Check sheet for the modelled part. Datum: model origin and axes. Units: mm. Face numbers are marked on the shaded views. A direction names the side the tool comes from. Give positions to 0.01 mm unless a question says otherwise; leave off trailing zeros. Order: outer loops, then holes, each group sorted by start corner. A loop starts at its lowest first (then second) coordinate and runs counter-clockwise, first axis right, second up. Notation, with made-up numbers: M 21.5,17 L 57.5,17 A11 ccw 57.5,32 Z; hole C 62,64.25 d8. An arc over 180 degrees is marked long. Return JSON: item names as keys, results as strings. Group by question number.
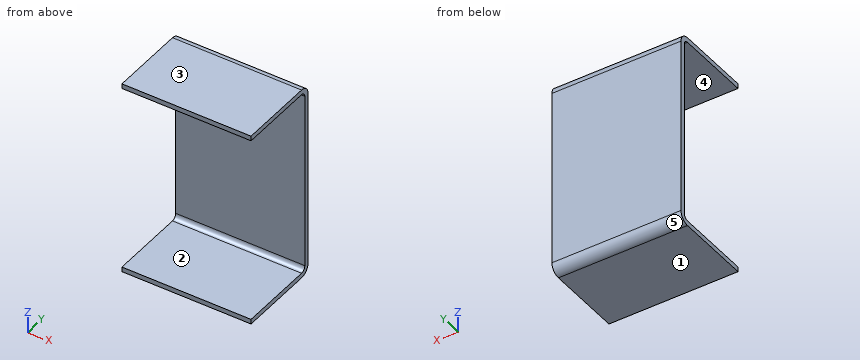
from build123d import *

# Parameters (mm, degrees)
EXTRUDE_1_DEPTH       = 40
SHEET_START           = -40
SHEET_METAL_1_DEPTH   = 80
SHEET_METAL_1_2_DEPTH = 80


# Read off the part's stored shape, not the designer's step: Преобразовать-Твердое тело1
with BuildPart() as part:
    # Sketch 1 → Вытянуть-Тонкостенный1 (new, symmetric)
    with BuildSketch(Plane(origin=(0, 0, 0), x_dir=(0, 0, -1), z_dir=(1, 0, 0))):
        Polygon((-58, -25), (-58, 25), (58, 25), (58, -25), (64, -25), (64, 31), (-64, 31), (-64, -25), align=None)
    extrude(amount=EXTRUDE_1_DEPTH, both=True)

    # Sheet Metal 1 outline → Sheet Metal 1 (cut)
    with BuildSketch(Plane.YZ.offset(SHEET_START)):
        with BuildLine():
            Line((-25, 64), (-25, 61))
            Line((-25, 61), (22, 61))
            ThreePointArc((22, 61), (26.242640687, 59.242640687), (28, 55))
            Line((28, 55), (28, -55))
            ThreePointArc((28, -55), (26.242640687, -59.242640687), (22, -61))
            Line((22, -61), (-25, -61))
            Line((-25, -61), (-25, -64))
            Line((-25, -64), (31, -64))
            Line((31, -64), (31, 64))
            Line((31, 64), (-25, 64))
        make_face()
    extrude(amount=SHEET_METAL_1_DEPTH, mode=Mode.SUBTRACT)

    # Sheet Metal 1 2 outline → Sheet Metal 1 2 (add)
    with BuildSketch(Plane.YZ.offset(SHEET_START)):
        with BuildLine():
            ThreePointArc((22, 58), (24.121320344, 57.121320344), (25, 55))
            Line((25, 55), (25, 58))
            Line((25, 58), (22, 58))
        make_face()
        with BuildLine():
            Line((25, -58), (25, -55))
            ThreePointArc((25, -55), (24.121320344, -57.121320344), (22, -58))
            Line((22, -58), (25, -58))
        make_face()
    extrude(amount=SHEET_METAL_1_2_DEPTH)


solid = part.part
1) Material ranges on line 1 along Z through (x, y) = (17, -18); line 2 along Y through (x, z) = (-11.5, -44); line 3 along Z through (x, y) = (-33.5, 26.5), recorded low to high.
2) Tool access check on the marked faces 4 and 5. Record the directions out of +Z, -Z, +X, -X, +Y, -Y that give a thin tool (end or side, any length) a straight path to the whole face; none if there is none.
3) Sectioned sample at A-A on y = -1.5. Record the boundary of the cut face in (x, z).
4) Sectioned sample at B-B on x = 5. Record the boundary of the cut face in (y, z), then the cut area to 3 significant figures.
5) Release check for a two-part mould opening along Z. For the marked faces 1, 2 and 3 record: released by +Z, released by -Z, zero draft, split by the parting line, or undercut.
6) Sectioned sample at C-C on z = -25.5. Record the boundary of the cut face in (x, y), then the cut area to 3 significant figures.
Reply:
{
 "1": {"line 1": "-61 to -58, 58 to 61", "line 2": "25 to 28", "line 3": "-58.97 to 58.97"},
 "2": {"face 4": "+X, -X, -Y", "face 5": "-Z, +X, -X, +Y"},
 "3": {"outline": "M -40,-61 L 40,-61 L 40,-58 L -40,-58 Z; M -40,58 L 40,58 L 40,61 L -40,61 Z"},
 "4": {"outline": "M -25,-61 L 22,-61 A6 ccw 28,-55 L 28,55 A6 ccw 22,61 L -25,61 L -25,58 L 22,58 A3 cw 25,55 L 25,-55 A3 cw 22,-58 L -25,-58 Z", "area": "654 mm^2"},
 "5": {"face 1": "released by -Z", "face 2": "undercut", "face 3": "released by +Z"},
 "6": {"outline": "M -40,25 L 40,25 L 40,28 L -40,28 Z", "area": "240 mm^2"}
}
